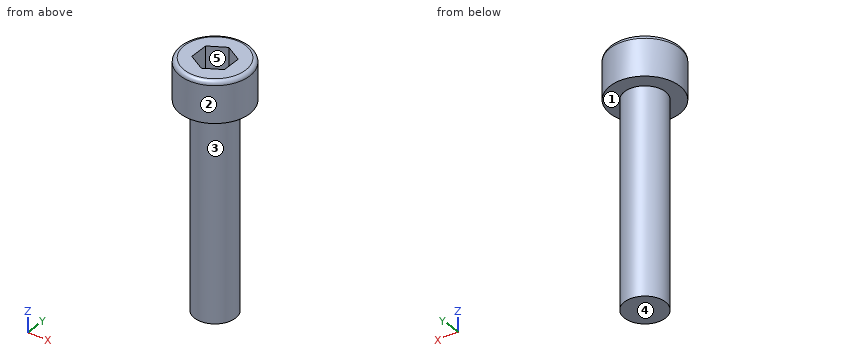
```python
from build123d import *

# Parameters (mm, degrees)
F0_R     = 4.25
F0_R_2   = 2.5
F1_DEPTH = 5
F2_DEPTH = 30
F3_DEPTH = 3
F4_R     = 0.5


with BuildPart() as f1:
    # F0 (on Top) → F1 (new body)
    with BuildSketch(Plane.XY):
        Circle(F0_R)
        Circle(F0_R_2, mode=Mode.SUBTRACT)
    extrude(amount=-F1_DEPTH)

    # F0 (on Top) → F2 (join)
    with BuildSketch(Plane.XY):
        Circle(F0_R_2)
        Polygon((0, 2.309401), (2, 1.154701), (2, -1.154701), (0, -2.309401), (-2, -1.154701), (-2, 1.154701), align=None, mode=Mode.SUBTRACT)
        Polygon((2, -1.154701), (2, 1.154701), (0, 2.309401), (-2, 1.154701), (-2, -1.154701), (0, -2.309401), align=None)
    extrude(amount=-F2_DEPTH)

    # F0 (on Top) → F3 (cut)
    with BuildSketch(Plane.XY):
        Polygon((2, -1.154701), (2, 1.154701), (0, 2.309401), (-2, 1.154701), (-2, -1.154701), (0, -2.309401), align=None)
    extrude(amount=-F3_DEPTH, mode=Mode.SUBTRACT)

    # F4
    f4_edges = [f1.edges().sort_by_distance(p)[0] for p in [
        (-4.25, 0, 0),
    ]]
    fillet(f4_edges, radius=F4_R)


solid = f1.part
```
Verification items for the finished model (mm, model axes). Face numbers are marked on the shaded views. A direction names the side the tool comes from. Give positions to 0.01 mm unless a question says otherwise; leave off trailing zeros. Write each loop counter-clockwise with the first axis right and the second up, starting at its lowest first coordinate (ties: lowest second). Pieces come first, ordered by that corner, then holes. Notation, with made-up numbers: (72.25, -8.5) - (127.25, -8.5) arc R25 ccw to (127.25, 7.5) - close; hole circle Ø7 at (17.25, 44.5). An arc over 180 degrees is marked (long way). Put each result on its own line as item: value.
Q1. Set-up check for the marked faces 1 and 2: record each of +Z, -Z, +X, -X, +Y, -Y from which the full face is reachable in a straight line by a thin tool's end or side.
Result:
face 1: -Z
face 2: +Z, -Z
Q2. Mould release check, pull along X, two halves, no side actions. Record for the marked faces 3, 4 and 5: released by +X, released by -X, zero draft, split by the parting line, or undercut.
Result:
face 3: split by the parting line
face 4: zero draft
face 5: undercut
Q3. Section check A-A on y = 0. Record the cut outline in (x, z), and give its area (3 significant figures).
Result:
outline: (-4.25, -5) - (-2.5, -5) - (-2.5, -30) - (2.5, -30) - (2.5, -5) - (4.25, -5) - (4.25, -0.5) arc R0.5 ccw to (3.75, 0) - (2, 0) - (2, -3) - (-2, -3) - (-2, 0) - (-3.75, 0) arc R0.5 ccw to (-4.25, -0.5) - close
area: 155 mm2
Q4. Scan lines: probe 1 along Z at (x, y) = (-3.5, 1.5); probe 2 along Z at (x, y) = (-0.75, 1.5); probe 3 along Y at (x, z) = (0, -17). Record each from-to range of solid material in increasing order. Write a range as from..to.
Result:
probe 1: -5..0
probe 2: -30..-3
probe 3: -2.5..2.5
Q5. Section check B-B on z = -17.25. Record the cut outline in (x, y), and give its area (3 significant figures).
Result:
outline: circle Ø5 at (0, 0)
area: 19.6 mm2
Q6. Depth check by flat-ended pin: P1, Ø1.5, axis at y = -1, z = -21.5, coming from the -X side; P2, Ø1.5, axis at x = 1, z = -18, coming from the -Y side; P3, Ø2, axis at x = 0, y = 1, coming from the +Z side. Enter the tip coordinate at first touch or a pass-through.
Result:
P1: x = -2.49
P2: y = -2.49
P3: z = -3
